```python
from build123d import *

# Parameters (mm, degrees)
F0_W     = 27
F0_H     = 24
F0_W_2   = 25
F0_H_2   = 22
F1_DEPTH = 60
F2_DEPTH = 1
F3_SIZE  = 1
F5_DEPTH = 25


with BuildPart() as f1:
    # F0 (on Front) → F1 (new body)
    with BuildSketch(Plane.XZ):
        with Locations((12.5, -11)):
            Rectangle(F0_W, F0_H)
        with Locations((12.5, -11)):
            Rectangle(F0_W_2, F0_H_2, mode=Mode.SUBTRACT)
    extrude(amount=F1_DEPTH)

    # F0 (on Front) → F2 (join)
    with BuildSketch(Plane.XZ):
        with Locations((12.5, -11)):
            Rectangle(F0_W, F0_H)
        with Locations((12.5, -11)):
            Rectangle(F0_W_2, F0_H_2, mode=Mode.SUBTRACT)
        with Locations((12.5, -11)):
            Rectangle(F0_W_2, F0_H_2)
    extrude(amount=-F2_DEPTH)

    # F3
    f3_edges = [f1.edges().sort_by_distance(p)[0] for p in [
        (0, -30, 0),
        (12.5, 0, 0),
        (0, 0, -11),
        (0, -30, -22),
        (12.5, 0, -22),
        (25, -30, -22),
        (25, 0, -11),
        (25, -30, 0),
        (-1, -29.5, 1),
        (-1, -29.5, -23),
        (-1, 1, -11),
        (26, -29.5, -23),
        (26, -29.5, 1),
        (12.5, 1, -23),
        (26, 1, -11),
        (12.5, 1, 1),
    ]]
    chamfer(f3_edges, length=F3_SIZE)

    # F4 (on face) → F5 (cut)
    with BuildSketch(Plane(origin=(0, 1, 0), x_dir=(-1, 0, 0), z_dir=(0, 1, 0))):
        Polygon((-19.20536533, -11), (-19.20536533, -13), (-5.20536533, -13), (-5.20536533, -9), (-19.20536533, -9), align=None)
    extrude(amount=-F5_DEPTH, mode=Mode.SUBTRACT)


solid = f1.part
```
CAD build for the part. Positions are in the model's coordinates, mm. A direction names the side the tool comes from. Round coordinates to 2 decimals unless told otherwise and drop trailing zeros. Write each loop counter-clockwise with the first axis right and the second up, starting at its lowest first coordinate (ties: lowest second). Pieces come first, ordered by that corner, then holes. Notation, with made-up numbers: (77.5, -35.5) - (94.5, -35.5) arc R24 cw to (94.5, 1.5) - close; hole circle Ø8 at (3, 87). An arc over 180 degrees is marked (long way). Return JSON: item names as keys, results as strings. Group by question number.
Item 1: Flat gauge pins, fed straight in: pin 1 Ø0.8 at (y, z) = (0.5, -10.5) entering from +X; pin 2 Ø0.5 at (y, z) = (0.5, -11) entering from -X; pin 3 Ø0.8 at (x, y) = (9.5, 0.5) entering from +Z. Where does each tip first touch, or does it go through?
Item 2: Probe probe 1 along X at (y, z) = (-22, -4.25); probe 2 along Z at (x, y) = (3.5, -50); probe 3 along Y at (x, z) = (15, -15). List the from-to ranges inside material, lowest first.
Item 3: Band-saw the part on D-D on x = 16.5. List the corners of the cut face in (y, z).
Item 4: Band-saw the part on B-B on x = 20. List the corners of the cut face in (y, z), plus the area to 3 significant figures.
Item 5: Band-saw the part on C-C on y = -22.5. List the corners of the cut face in (x, z), plus the area to 3 significant figures.
Item 6: 3-axis set-ups, long thin cutter, end or side, ignore diameter. For faces 1 (the face through (12, 1, -8)), 2 (the face through (25, -30, -11)): which of +Z, -Z, +X, -X, +Y, -Y reach the whole face in a straight line?
Item 7: Mould opens along X. For faces 3 (the face through (26, -30, -11)), 4 (the face through (-1, -30, -11)), 5 (the face through (12, -30, 0)), 6 (the face through (12, -30, 1)) say: +X half, -X half, draft (parallel to the pull), parting line (faces both ways), or undercut.
Item 8: Band-saw the part on A-A on z = -9.75. List the corners of the cut face in (x, y), plus the area to 3 significant figures.
Resolved:
{
 "1": {"pin 1": "stops at x = 25.9", "pin 2": "stops at x = -0.75", "pin 3": "stops at z = 0.9"},
 "2": {"probe 1": "x = -1 to 0, 25 to 26", "probe 2": "z = -23 to -22, 0 to 1", "probe 3": "y = 0 to 1"},
 "3": {"outline": "(-60, -23) - (0, -23) - (1, -22) - (1, -13) - (0, -13) - (0, -21) - (-1, -22) - (-60, -22) - close; (-60, 0) - (-1, 0) - (0, -1) - (0, -9) - (1, -9) - (1, 0) - (0, 1) - (-60, 1) - close"},
 "4": {"outline": "(-60, -23) - (0, -23) - (1, -22) - (1, 0) - (0, 1) - (-60, 1) - (-60, 0) - (-1, 0) - (0, -1) - (0, -21) - (-1, -22) - (-60, -22) - close", "area": "144 mm²"},
 "5": {"outline": "(-1, -22) - (0, -23) - (25, -23) - (26, -22) - (26, 0) - (25, 1) - (0, 1) - (-1, 0) - close; hole (0, -21) - (1, -22) - (24, -22) - (25, -21) - (25, -1) - (24, 0) - (1, 0) - (0, -1) - close", "area": "98.0 mm²"},
 "6": {"face 1": "+Z, -Z, +X, -X, +Y", "face 2": "-Y"},
 "7": {"face 3": "+X half", "face 4": "-X half", "face 5": "undercut", "face 6": "draft"},
 "8": {"outline": "(-1, -60) - (0, -60) - (0, -1) - (1, 0) - (5.21, 0) - (5.21, 1) - (0, 1) - (-1, 0) - close; (19.21, 0) - (24, 0) - (25, -1) - (25, -60) - (26, -60) - (26, 0) - (25, 1) - (19.21, 1) - close", "area": "133 mm²"}
}
